Geometry: see drawing. Coordinates: mm, zero at the bounding-box minimum. Round coordinates to 2 decimals unless told otherwise and drop trailing zeros. Write each loop counter-clockwise with the first axis right and the second up, starting at its lowest first coordinate (ties: lowest second). Pieces come first, ordered by that corner, then holes. Notation, with made-up numbers: M 25,80.5 L 71,80.5 A17 ccw 71,92.5 Z; hole C 13,70.25 d5. An arc over 180 degrees is marked long. Use a Markdown table: item, result.
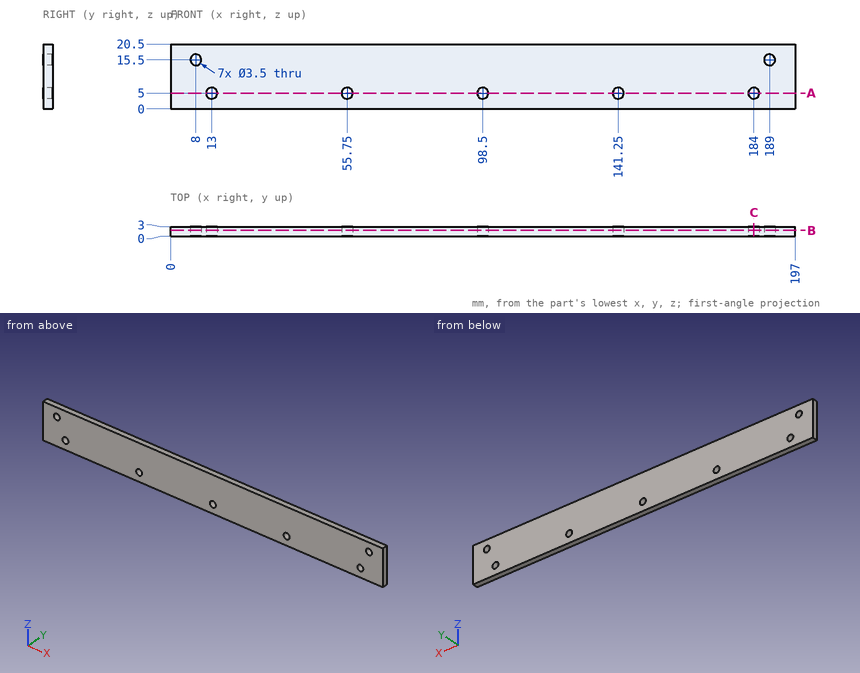
Q1. Section A-A on z = 5. Return loops of the section in (x, y).
Results are:
| item | result |
|---|---|
| outline | M 0,0 L 11.25,0 L 11.25,3 L 0,3 Z; M 14.75,0 L 54,0 L 54,3 L 14.75,3 Z; M 57.5,0 L 96.75,0 L 96.75,3 L 57.5,3 Z; M 100.25,0 L 139.5,0 L 139.5,3 L 100.25,3 Z; M 143,0 L 182.25,0 L 182.25,3 L 143,3 Z; M 185.75,0 L 197,0 L 197,3 L 185.75,3 Z |
Q2. Section C-C on x = 184. Return loops of the section in (y, z).
Results are:
| item | result |
|---|---|
| outline | M 0,0 L 3,0 L 3,3.25 L 0,3.25 Z; M 0,6.75 L 3,6.75 L 3,20.5 L 0,20.5 Z |
Q3. Line query: L1, parallel to X at y = 2, z = 5; L2, parallel to X at y = 2, z = 15.5; L3, parallel to Z at x = 141.25, y = 1.7. Output: solid intervals per line, ascending.
Results are:
| item | result |
|---|---|
| L1 | 0 to 11.25, 14.75 to 54, 57.5 to 96.75, 100.25 to 139.5, 143 to 182.25, 185.75 to 197 |
| L2 | 0 to 6.25, 9.75 to 187.25, 190.75 to 197 |
| L3 | 0 to 3.25, 6.75 to 20.5 |
Q4. First-contact query: pin 1 Ø5.5 at (x, z) = (98.5, 5) entering from -Y; pin 2 Ø3 at (x, z) = (141.25, 5) entering from -Y. Flat tips, straight axial feed; report the tip coordinate or a pass-through.
Results are:
| item | result |
|---|---|
| pin 1 | y = 0 |
| pin 2 | through |
Q5. Section B-B on y = 1.95. Return loops of the section in (x, z).
Results are:
| item | result |
|---|---|
| outline | M 0,0 L 197,0 L 197,20.5 L 0,20.5 Z; hole C 8,15.5 d3.5; hole C 13,5 d3.5; hole C 55.75,5 d3.5; hole C 98.5,5 d3.5; hole C 141.25,5 d3.5; hole C 184,5 d3.5; hole C 189,15.5 d3.5 |
